Verification items for the finished model (mm, model axes). Face numbers are marked on the shaded views. A direction names the side the tool comes from. Round coordinates to 2 decimals unless told otherwise and drop trailing zeros. Write each loop counter-clockwise with the first axis right and the second up, starting at its lowest first coordinate (ties: lowest second). Pieces come first, ordered by that corner, then holes.
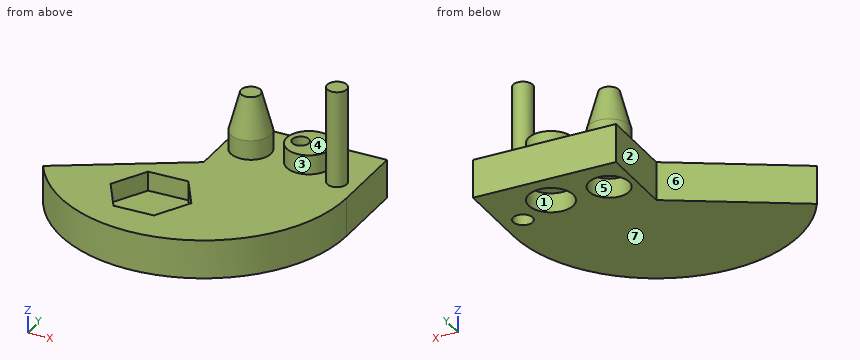
from build123d import *

# Parameters (mm, degrees)
F0_R      = 13.1789496922
F1_DEPTH  = 25.4
F0_R_2    = 14.6674866232
F0_R_3    = 5.4973214865
F0_W      = 94.0474122763
F0_H      = 51.4852851629
F0_R_4    = 6.4238066615
F2_DEPTH  = 12.7
F3_DEPTH  = 76.2
F1_FACE_R = 13.1789496922
F4_DEPTH  = 25.4
F4_TAPER  = 15
F2_FACE_W = 94.0474122763
F2_FACE_H = 25.4
F5_ANGLE  = 150
F7_DEPTH  = 12.7


with BuildPart() as f1:
    # F0 (on Top) → F1 (new body)
    with BuildSketch(Plane.XY):
        with Locations((17.2175206244, 26.8186014146)):
            Circle(F0_R)
    extrude(amount=F1_DEPTH)



with BuildPart() as f1b:
    # F0 (on Top) → F1, piece 2 (new body)
    with BuildSketch(Plane.XY):
        with Locations((54.7939687967, 28.1190406531)):
            Circle(F0_R_2)
        with Locations((49.2966473103, 28.1190406531)):
            Circle(F0_R_3, mode=Mode.SUBTRACT)
    extrude(amount=F1_DEPTH)


with BuildPart() as f1_1:
    add(f1.part)

    add(f1b.part)  # F2 merges F1b
    # F0 (on Top) → F2 (join, symmetric)
    with BuildSketch(Plane.XY):
        with Locations((47.0237061381, 25.7426425815)):
            Rectangle(F0_W, F0_H)
        with Locations((80.1606476307, 14.6344061941)):
            Circle(F0_R_4, mode=Mode.SUBTRACT)
        with Locations((17.2175206244, 26.8186014146)):
            Circle(F0_R, mode=Mode.SUBTRACT)
        with Locations((54.7939687967, 28.1190406531)):
            Circle(F0_R_2, mode=Mode.SUBTRACT)
    extrude(amount=F2_DEPTH, both=True)

    # F0 (on Top) → F3 (join)
    with BuildSketch(Plane.XY):
        with Locations((80.1606476307, 14.6344061941)):
            Circle(F0_R_4)
    extrude(amount=F3_DEPTH)

    # F1_face (on face) → F4 (join)
    with BuildSketch(Plane(origin=(17.2175206244, 26.8186014146, 25.4), x_dir=(1, 0, 0), z_dir=(0, 0, 1))):
        Circle(F1_FACE_R)
    extrude(amount=F4_DEPTH, taper=F4_TAPER)

    # F2_face (on face) → F5 (revolve)
    with BuildSketch(Plane(origin=(47.0237061381, 0, 0), x_dir=(1, 0, 0), z_dir=(0, -1, 0))):
        Rectangle(F2_FACE_W, F2_FACE_H)
    revolve(axis=Axis((0, 0, 0), (0, 0, -1)), revolution_arc=F5_ANGLE)

    # F6 (on face) → F7 (cut)
    with BuildSketch(Plane.XY.offset(12.7)):
        Polygon((16.165189955, -47.1866849835), (2.6281359163, -24.5952483242), (-23.705149158, -25.0229626845), (-36.5013801936, -48.042113704), (-22.9643261549, -70.6335503633), (3.3689589194, -70.205836003), align=None)
    extrude(amount=-F7_DEPTH, mode=Mode.SUBTRACT)


solid = f1_1.part
Q1. Tool access check on the marked faces 1, 2 and 3. Record the directions out of +Z, -Z, +X, -X, +Y, -Y that give a thin tool (end or side, any length) a straight path to the whole face; none if there is none.
Recorded:
face 1: -Z
face 2: +Z, -Z, -X, +Y
face 3: +Z
Q2. Sectioned sample at A-A (x = 51). Enter the section's corners in (y, z), plus the area to 3 significant figures.
Recorded:
outline: (-79.02, -12.7) - (13.95, -12.7) - (13.95, 0) - (22.89, 0) - (22.89, 25.4) - (13.95, 25.4) - (13.95, 12.7) - (-79.02, 12.7) - close; (33.35, 0) - (42.29, 0) - (42.29, -12.7) - (51.49, -12.7) - (51.49, 12.7) - (42.29, 12.7) - (42.29, 25.4) - (33.35, 25.4) - close
area: 3,050 mm2
Q3. Release check for a two-part mould opening along X. For the marked faces 4, 5, 6 and 7 record: released by +X, released by -X, zero draft, split by the parting line, or undercut.
Recorded:
face 4: undercut
face 5: undercut
face 6: released by -X
face 7: zero draft
Q4. Sectioned sample at B-B (z = 41). Enter the section's corners in (x, y).
Recorded:
outline: circle Ø18 at (17.22, 26.82); circle Ø12.85 at (80.16, 14.63)
Q5. Sectioned sample at D-D (x = -12.5). Enter the section's corners in (y, z).
Recorded:
outline: (-93.21, -12.7) - (-7.22, -12.7) - (-7.22, 12.7) - (-24.84, 12.7) - (-24.84, 0) - (-70.46, 0) - (-70.46, 12.7) - (-93.21, 12.7) - close
Q6. Material ranges on line 1 along Z through (x, y) = (55.5, 26.5); line 2 along X through (y, z) = (38, 11.5); line 3 along X through (y, z) = (17, -5), recorded low to high.
Recorded:
line 1: z = 0 to 25.4
line 2: x = 0 to 94.05
line 3: x = 0 to 8.43, 26.01 to 45.23, 64.36 to 74.19, 86.13 to 94.05
Q7. Sectioned sample at C-C (y = -57). Enter the section's corners in (x, z).
Recorded:
outline: (-74.81, -12.7) - (74.81, -12.7) - (74.81, 12.7) - (10.71, 12.7) - (10.71, 0) - (-31.13, 0) - (-31.13, 12.7) - (-74.81, 12.7) - close
Q8. Depth check by flat-ended pin: P1, Ø8, axis at x = 54, y = 30, coming from the +Z side; P2, Ø8, axis at x = 16.5, y = 21, coming from the -Z side; P3, Ø4, axis at x = 17, y = -8.5, coming from the +Z side. Enter the tip coordinate at first touch or a pass-through.
Recorded:
P1: stops at z = 25.4
P2: stops at z = 0
P3: stops at z = 12.7
